The listing builds one solid part. Answer for the finished solid, in the listing's coordinates (mm). Face numbers are marked on the shaded views. A direction names the side the tool comes from. Give positions to 0.01 mm unless a question says otherwise; leave off trailing zeros. Order: outer loops, then holes, each group sorted by start corner. A loop starts at its lowest first (then second) coordinate and runs counter-clockwise, first axis right, second up. Notation, with made-up numbers: (71, -7) - (84, -7) arc R24 ccw to (84, 19) - close; hole circle Ø11 at (32.5, 24.25). An arc over 180 degrees is marked (long way). Answer in a Markdown table with one row per item. Add a question column.
```python
from build123d import *

# Parameters (mm, degrees)
PAD013_DEPTH    = 2
PAD014_DEPTH    = 1.2
SKETCH061_R     = 2
POCKET010_DEPTH = 3.201
CHAMFER009_SIZE = 1


with BuildPart() as part:
    # Sketch034 → Pad013 (new body)
    with BuildSketch(Plane.XZ):
        with BuildLine():
            ThreePointArc((-7.12, 25), (-9.24132, 24.12132), (-10.12, 22))
            Line((-10.12, 22), (-10.12, 2))
            Line((-10.12, 2), (-12.12, -2))
            ThreePointArc((-12.12, -2), (-14.24132, -2.87868), (-15.12, -5))
            Line((-15.12, -5), (-15.12, -19))
            ThreePointArc((-15.12, -19), (-14.24132, -21.12132), (-12.12, -22))
            Line((-12.12, -22), (12.12, -22))
            ThreePointArc((12.12, -22), (14.24132, -21.12132), (15.12, -19))
            Line((15.12, -19), (15.12, -5))
            ThreePointArc((15.12, -5), (14.24132, -2.87868), (12.12, -2))
            Line((10.12, 2), (12.12, -2))
            Line((10.12, 22), (10.12, 2))
            ThreePointArc((10.12, 22), (9.24132, 24.12132), (7.12, 25))
            Line((-7.12, 25), (7.12, 25))
        make_face()
        with BuildLine():
            Line((-3.5, 18.88), (3.5, 18.88))
            ThreePointArc((4, 18.38), (3.853553, 18.733553), (3.5, 18.88))
            Line((4, 18.38), (4, 11.38))
            ThreePointArc((3.5, 10.88), (3.853553, 11.026447), (4, 11.38))
            Line((3.5, 10.88), (-3.5, 10.88))
            ThreePointArc((-4, 11.38), (-3.853553, 11.026447), (-3.5, 10.88))
            Line((-4, 11.38), (-4, 18.38))
            ThreePointArc((-3.5, 18.88), (-3.853553, 18.733553), (-4, 18.38))
        make_face(mode=Mode.SUBTRACT)
    extrude(amount=PAD013_DEPTH)

    # Sketch035 → Pad014 (join)
    with BuildSketch(Plane.XZ.offset(2)):
        with BuildLine():
            ThreePointArc((15.12, -5), (14.24132, -2.87868), (12.12, -2))
            Line((-12.12, -2), (12.12, -2))
            ThreePointArc((-12.12, -2), (-14.24132, -2.87868), (-15.12, -5))
            Line((-15.12, -19), (-15.12, -5))
            ThreePointArc((-15.12, -19), (-14.24132, -21.12132), (-12.12, -22))
            Line((12.12, -22), (-12.12, -22))
            ThreePointArc((12.12, -22), (14.24132, -21.12132), (15.12, -19))
            Line((15.12, -5), (15.12, -19))
        make_face()
    extrude(amount=PAD014_DEPTH)

    # Sketch061 → Pocket010 (cut, through all)
    with BuildSketch(Plane.XZ):
        with Locations((-10.705786, -17.585786)):
            Circle(SKETCH061_R)
        with Locations((10.705786, -17.585786)):
            Circle(SKETCH061_R)
    extrude(amount=POCKET010_DEPTH, mode=Mode.SUBTRACT)

    # Chamfer009
    chamfer009_edges = [part.edges().sort_by_distance(p)[0] for p in [
        (-12.705786, 0, -17.585786),
        (-8.705786, -1.6, -17.585786),
        (-12.705786, -3.2, -17.585786),
        (8.705786, 0, -17.585786),
        (12.705786, -1.6, -17.585786),
        (8.705786, -3.2, -17.585786),
    ]]
    chamfer(chamfer009_edges, length=CHAMFER009_SIZE)


solid = part.part
```
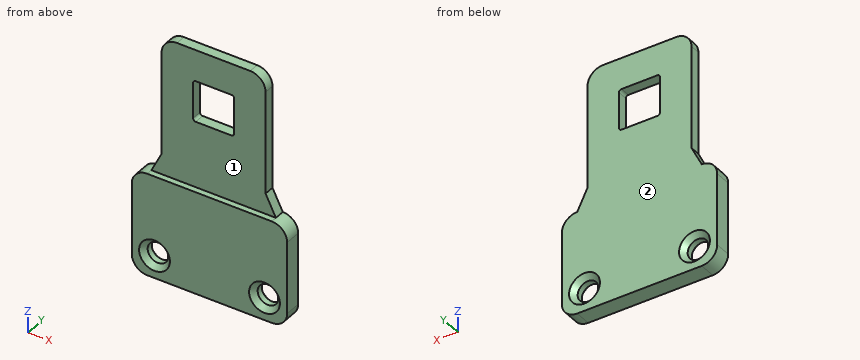
(1) Straight lines are drawn through the part: line 1 (X direction, y = -1.4, z = -17.5); line 2 (X direction, y = -3, z = -15.5); line 3 (Z direction, x = -1, y = -1.35). For each, find the intervals that lie inside material, in ascending order.
(2) Find section B-B, the plane z = 10. Write down the section's boundary in (x, y).
(3) Find section A-A, the plane x = -1. Write down the section's boundary in (y, z), plus the area to 3 significant figures.
(4) Each of these flat-tipped pins is pushed along its axis until it touches: P1, Ø1.6, axis at y = -1, z = 10.5, coming from the -X side; P2, Ø1, axis at x = 1, y = -3, coming from the +Z side; P3, Ø1, axis at y = -1, z = 8.5, coming from the +X side; P4, Ø3.5, axis at x = 10.71, z = -17.59, coming from the -Y side. Where does it stop, or does it pass through?
(5) For the marked faces 1 and 2, determine the directions among +Z, -Z, +X, -X, +Y, -Y from which every point of the face is accessible in a straight line to the end or side of a thin tool.
Answer key:
| question | item | result |
|---|---|---|
| 1 | line 1 | -15.12 to -12.7, -8.71 to 8.71, 12.7 to 15.12 |
| 1 | line 2 | -15.12 to -12.57, -8.84 to 8.84, 12.57 to 15.12 |
| 1 | line 3 | -22 to 10.88, 18.88 to 25 |
| 2 | outline | (-10.12, -2) - (10.12, -2) - (10.12, 0) - (-10.12, 0) - close |
| 3 | outline | (-3.2, -22) - (0, -22) - (0, 10.88) - (-2, 10.88) - (-2, -2) - (-3.2, -2) - close; (-2, 18.88) - (0, 18.88) - (0, 25) - (-2, 25) - close |
| 3 | area | 102 mm² |
| 4 | P1 | x = -10.12 |
| 4 | P2 | z = -2 |
| 4 | P3 | x = 10.12 |
| 4 | P4 | through |
| 5 | face 1 | +Z, +X, -X, -Y |
| 5 | face 2 | +Z, -Z, +X, -X, +Y |
